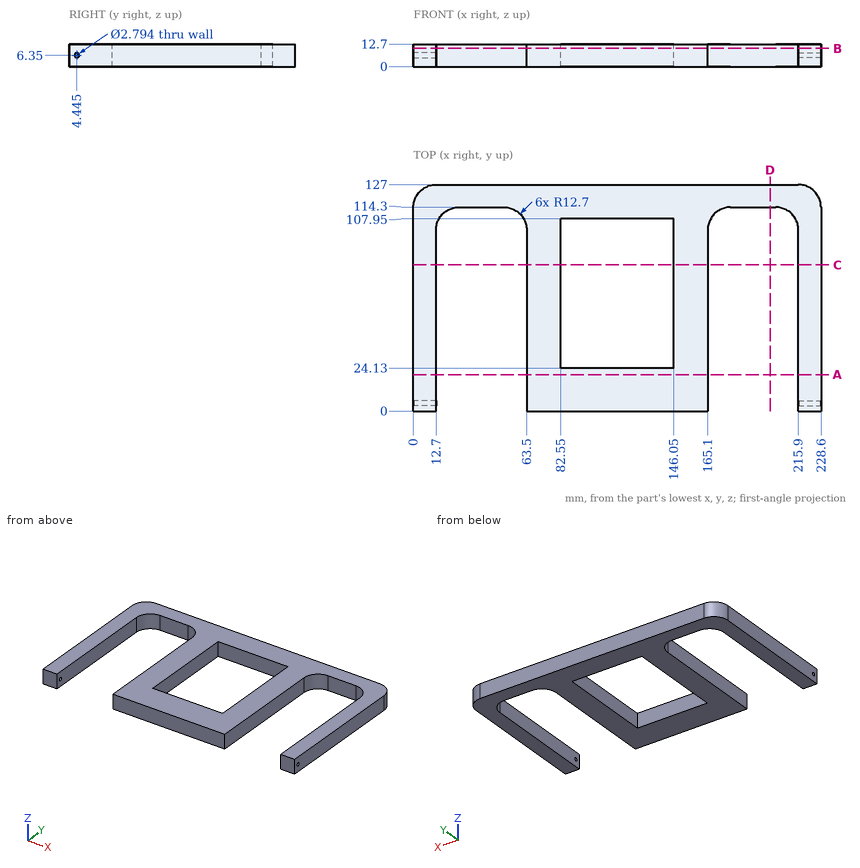
Verification items for this drawing (mm, ordinates from the low corner). Give positions to 0.01 mm unless a question says otherwise; leave off trailing zeros. Write each loop counter-clockwise with the first axis right and the second up, starting at its lowest first coordinate (ties: lowest second). Pieces come first, ordered by that corner, then holes. Notation, with made-up numbers: (-27.5, -2.75) -> (23.5, -2.75) arc R34 cw to (23.5, 31.25) -> close; hole circle Ø9 at (60, 80). An arc over 180 degrees is marked (long way). Write item = value, one per line.
Item 1: Gauge pin test, flat ends, axial feed: pin 1 (4 mm diameter, centred on x = 195, z = 6.5, fed in from -Y); pin 2 (1.5 mm diameter, centred on y = 23.5, z = 4.5, fed in from -X); pin 3 (2.5 mm diameter, centred on y = 4.445, z = 6.35, fed in from +X). Record the tip position at first contact, or that the pin passes through.
Output:
pin_1 = 114.3
pin_2 = 0
pin_3 = 165.1
Item 2: Sectioned sample at A-A on y = 20.5. Record the boundary of the cut face in (x, z).
Output:
outline = (0, 0) -> (12.7, 0) -> (12.7, 12.7) -> (0, 12.7) -> close; (63.5, 0) -> (165.1, 0) -> (165.1, 12.7) -> (63.5, 12.7) -> close; (215.9, 0) -> (228.6, 0) -> (228.6, 12.7) -> (215.9, 12.7) -> close
Item 3: Sectioned sample at C-C on y = 82. Record the boundary of the cut face in (x, z).
Output:
outline = (0, 0) -> (12.7, 0) -> (12.7, 12.7) -> (0, 12.7) -> close; (63.5, 0) -> (82.55, 0) -> (82.55, 12.7) -> (63.5, 12.7) -> close; (146.05, 0) -> (165.1, 0) -> (165.1, 12.7) -> (146.05, 12.7) -> close; (215.9, 0) -> (228.6, 0) -> (228.6, 12.7) -> (215.9, 12.7) -> close
Item 4: Scan lines: probe 1 along X at (y, z) = (37.5, 3); probe 2 along Y at (x, z) = (91.5, 4.5); probe 3 along X at (y, z) = (6, 0.5). Record each from-to range of solid material in increasing order. Write a range as from..to.
Output:
probe_1 = 0..12.7, 63.5..82.55, 146.05..165.1, 215.9..228.6
probe_2 = 0..24.13, 107.95..127
probe_3 = 0..12.7, 63.5..165.1, 215.9..228.6
Item 5: Sectioned sample at D-D on x = 200. Record the boundary of the cut face in (y, z).
Output:
outline = (114.3, 0) -> (127, 0) -> (127, 12.7) -> (114.3, 12.7) -> close
Item 6: Sectioned sample at B-B on z = 10.25. Record the boundary of the cut face in (x, y).
Output:
outline = (0, 0) -> (12.7, 0) -> (12.7, 101.6) arc R12.7 cw to (25.4, 114.3) -> (50.8, 114.3) arc R12.7 cw to (63.5, 101.6) -> (63.5, 0) -> (165.1, 0) -> (165.1, 101.6) arc R12.7 cw to (177.8, 114.3) -> (203.2, 114.3) arc R12.7 cw to (215.9, 101.6) -> (215.9, 0) -> (228.6, 0) -> (228.6, 114.3) arc R12.7 ccw to (215.9, 127) -> (12.7, 127) arc R12.7 ccw to (0, 114.3) -> close; hole (82.55, 24.13) -> (146.05, 24.13) -> (146.05, 107.95) -> (82.55, 107.95) -> close
